```python
from build123d import *

# Parameters (mm, degrees)
SKETCH_1_W      = 11.9
SKETCH_1_H      = 11.9
SKETCH_1_R      = 5.05
EXTRUDE_1_DEPTH = 2.8
CHAMFER_1_SIZE  = 0.9


with BuildPart() as part:
    # 草图1 → 凸台-拉伸1 (new body)
    with BuildSketch(Plane(origin=(0, 0, 0), x_dir=(1, 0, 0), z_dir=(0, 1, 0))):
        Rectangle(SKETCH_1_W, SKETCH_1_H)
        with Locations(Location((0, 0, 0), (0, 0, 270))):
            Circle(SKETCH_1_R, mode=Mode.SUBTRACT)
    extrude(amount=EXTRUDE_1_DEPTH)

    # 倒角1
    chamfer_1_edges = [part.edges().sort_by_distance(p)[0] for p in [
        (0, 2.8, -5.05),
    ]]
    chamfer(chamfer_1_edges, length=CHAMFER_1_SIZE - 0.0001)  # a hair under: the kernel refuses the full size


solid = part.part
```
Build history of the part. All positions in model axes, mm. Coordinates: 2 decimals unless noted, no trailing zeros. Order: outer loops, then holes, each group sorted by start corner. A loop starts at its lowest first (then second) coordinate and runs counter-clockwise, first axis right, second up.
Item 1: Drill centre lines: L1, parallel to X at y = 0.6, z = 0; L2, parallel to X at y = 2.6, z = 2.25; L3, parallel to Z at x = 2.5, y = 0.8. Where is each one in solid material? Low to high.
Filled in:
L1: x = -5.95 to -5.05, 5.05 to 5.95
L2: x = -5.95 to -5.29, 5.29 to 5.95
L3: z = -5.95 to -4.39, 4.39 to 5.95
Item 2: Mould opens along Z. For faces 1 (the flat face through (0, 1, -5.95)), 2 (the cylindrical face through (-3.07, 0.94, -4.01)), 3 (the flat face through (0, 1, 5.95)), 4 (the flat face through (-5.95, 1, 0)) say: released by +Z, released by -Z, zero draft, split by the parting line, or undercut.
Filled in:
face 1: released by -Z
face 2: undercut
face 3: released by +Z
face 4: zero draft
Item 3: Saw through at C-C on y = 1.7. List the corners of the cut face in (x, z).
Filled in:
outline: (-5.95, -5.95) - (5.95, -5.95) - (5.95, 5.95) - (-5.95, 5.95) - close; hole circle Ø10.1 at (0, 0)
Item 4: Drop a flat-ended pin along its axis: pin 1 Ø1.5 at (x, z) = (-3.5, -3) entering from +Y. Give the stop position or say it passes through.
Filled in:
pin 1: stops at y = 2.21
